```python
from build123d import *

# Parameters (mm, degrees)
BOSS_EXTRUDE2_DEPTH = 431.8
CUT_EXTRUDE3_DEPTH  = 127
SKETCH7_R           = 6.3881
CUT_EXTRUDE4_DEPTH  = 127


with BuildPart() as part:
    # Sketch3 → Boss-Extrude2 (new body)
    with BuildSketch(Plane.XY):
        Polygon((0, 0), (0, 49.2125), (-1.5875, 49.2125), (-1.5875, -1.5875), (49.2125, -1.5875), (49.2125, 0), align=None)
    extrude(amount=BOSS_EXTRUDE2_DEPTH)

    # Sketch6 → Cut-Extrude3 (cut)
    with BuildSketch(Plane(origin=(0, 0, 0), x_dir=(0, 0, -1), z_dir=(1, 0, 0))):
        with BuildLine():
            Line((-384.0054804, 31.187094829), (-244.3054804, 31.187094829))
            ThreePointArc((-244.3054804, 31.187094829), (-237.8919804, 24.773594829), (-244.3054804, 18.360094829))
            Line((-244.3054804, 18.360094829), (-384.0054804, 18.360094829))
            ThreePointArc((-384.0054804, 18.360094829), (-390.4189804, 24.773594829), (-384.0054804, 31.187094829))
        make_face()
    extrude(amount=-CUT_EXTRUDE3_DEPTH, mode=Mode.SUBTRACT)

    # Sketch7 → Cut-Extrude4 (cut)
    with BuildSketch(Plane(origin=(0, 0, 0), x_dir=(0, 0, -1), z_dir=(1, 0, 0))):
        with Locations(Location((-29.538792285, 24.773594829, 0), (0, 0, 90))):
            Circle(SKETCH7_R)
    extrude(amount=-CUT_EXTRUDE4_DEPTH, mode=Mode.SUBTRACT)


solid = part.part
```
Here's how the part is built. I have some questions about the finished solid (model axes, mm). A direction names the side the tool comes from. Round coordinates to 2 decimals unless told otherwise and drop trailing zeros. Write each loop counter-clockwise with the first axis right and the second up, starting at its lowest first coordinate (ties: lowest second). Pieces come first, ordered by that corner, then holes.
Q1. If we section it at B-B on y = 25.5: Write out the boundary of the cut face in (x, z), plus the area to 3 significant figures.
Q2. If we section it at C-C on z = 167.5: Write out the boundary of the cut face in (x, y).
Q3. Will these pins go through, and if not, where does the flat tip stop? P1, Ø2, axis at x = 37.5, z = 371, coming from the +Y side; P2, Ø8, axis at y = 14.5, z = 90.5, coming from the +X side.
Q4. Please list where this line runs through material, in increasing order: probe 1 along X at (y, z) = (47, 273).
Q5. If we section it at A-A on z = 299.5: Write out the boundary of the cut face in (x, y).
Q6. If we mould it in two halves opening along Y, with no side actions, what happens to faces 1 (the flat face through (23, -1.588, 213)), 2 (the flat face through (-1, 13, 431.8)), 3 (the flat face through (25, 0, 213)), 4 (the cylindrical face through (-0.78, 27.72, 23.87))? For each: +Y half, -Y half, draft (parallel to the pull), parting line (faces both ways), or undercut.
Q7. Which directions (+Z, -Z, +X, -X, +Y, -Y) give clear straight access to the entire face, cutting with the end or side of a thin tool? Please do faces 5 (the flat face through (0, 24, 213)), 6 (the flat face through (-1, 13, 0)).
Q8. If we section it at D-D on x = 31: Write out the boundary of the cut face in (y, z), plus the area to 3 significant figures.
Answer below:
1. outline: (-1.59, 0) - (0, 0) - (0, 23.19) - (-1.59, 23.19) - close; (-1.59, 35.89) - (0, 35.89) - (0, 237.93) - (-1.59, 237.93) - close; (-1.59, 390.38) - (0, 390.38) - (0, 431.8) - (-1.59, 431.8) - close
1. area: 423 mm2
2. outline: (-1.59, -1.59) - (49.21, -1.59) - (49.21, 0) - (0, 0) - (0, 49.21) - (-1.59, 49.21) - close
3. P1: stops at y = 0
3. P2: stops at x = 0
4. probe 1: x = -1.59 to 0
5. outline: (-1.59, -1.59) - (49.21, -1.59) - (49.21, 0) - (0, 0) - (0, 18.36) - (-1.59, 18.36) - close; (-1.59, 31.19) - (0, 31.19) - (0, 49.21) - (-1.59, 49.21) - close
6. face 1: -Y half
6. face 2: draft
6. face 3: +Y half
6. face 4: undercut
7. face 5: +Z, -Z, +X, +Y
7. face 6: -Z, +X, -X, +Y, -Y
8. outline: (-1.59, 0) - (0, 0) - (0, 431.8) - (-1.59, 431.8) - close
8. area: 685 mm2
